Build history of the part. All positions in model axes, mm. Face numbers are marked on the shaded views. A direction names the side the tool comes from. Give positions to 0.01 mm unless a question says otherwise; leave off trailing zeros. Loops run counter-clockwise (first coordinate to the right, second up) from the corner with the lowest first, then second, coordinate; pieces in that order, holes last. Notation, with made-up numbers: (82.25, -17.5) -> (141.25, -17.5) arc R26 ccw to (141.25, 3.5) -> close; hole circle Ø2 at (-32, 78). An arc over 180 degrees is marked (long way). Answer as a JSON object with one key per item and string values. Group by question number.
Q1. Band-saw the part on B-B, the plane z = 0. Write the cut outline in (x, y).
Q2. Drop flat-ended pins along their axis: pin 1 (4 mm diameter, centred on x = 1, y = 27, fed in from -Z); pin 2 (4 mm diameter, centred on x = -8, z = -1.5, fed in from +Y); pin 3 (2 mm diameter, centred on y = 14, z = 1.5, fed in from +X); pin 4 (2.5 mm diameter, centred on y = 14, z = 0.5, fed in from -X). Give the stop position or say it passes through.
Q3. Two-plate mould, pull along X, no slides. Class the marked faces 1, 2 and 3: pulls with the +X half, pulls with the -X half, needs draft (parallel to the pull), parting line crosses it, or undercut.
Q4. Tool access for the marked faces 4, 5 and 6: list every direction of +Z, -Z, +X, -X, +Y, -Y with a clear straight run to the whole face (end or side of a thin tool).
Q5. Band-saw the part on A-A, the plane x = 0. Write the cut outline in (y, z), plus the area to 3 significant figures.
Q6. Wall check: probe 1 along Z at (x, y) = (0, 40); probe 2 along X at (y, z) = (6.5, 7.75); probe 3 along Z at (x, y) = (-11.25, 15). Give the ranges that are in metal, low to high. Write a range as from..to.
from build123d import *

# Parameters (mm, degrees)
F1_DEPTH = 50.8
F2_R     = 2.6035
F3_DEPTH = 50.801


with BuildPart() as f1:
    # F0 (on Front) → F1 (new body)
    with BuildSketch(Plane.XZ):
        with BuildLine():
            Line((-4.5085, 0), (0, 0))
            Line((0, 0), (0, 4.5085))
            Line((0, 4.5085), (-2.54, 4.5085))
            ThreePointArc((-2.54, 4.5085), (-2.957967, 4.591639), (-3.312302, 4.828398))
            Line((-3.312302, 4.828398), (-7.109602, 8.625698))
            ThreePointArc((-7.109602, 8.625698), (-7.346361, 9.815967), (-6.3373, 10.4902))
            Line((-6.3373, 10.4902), (-4.3307, 10.4902))
            ThreePointArc((-4.3307, 10.4902), (-3.558398, 10.810098), (-3.2385, 11.5824))
            Line((-3.2385, 11.5824), (-3.2385, 11.6078))
            ThreePointArc((-3.2385, 11.6078), (-3.558398, 12.380102), (-4.3307, 12.7))
            Line((-4.3307, 12.7), (-11.6078, 12.7))
            ThreePointArc((-11.6078, 12.7), (-12.380102, 12.380102), (-12.7, 11.6078))
            Line((-12.7, 11.6078), (-12.7, 4.3434))
            ThreePointArc((-12.7, 4.3434), (-12.380102, 3.571098), (-11.6078, 3.2512))
            Line((-11.6078, 3.2512), (-11.5824, 3.2512))
            ThreePointArc((-11.5824, 3.2512), (-10.810098, 3.571098), (-10.4902, 4.3434))
            Line((-10.4902, 4.3434), (-10.4902, 6.244363))
            ThreePointArc((-10.4902, 6.244363), (-9.815967, 7.253424), (-8.625698, 7.016665))
            Line((-8.625698, 7.016665), (-4.828398, 3.219365))
            ThreePointArc((-4.828398, 3.219365), (-4.591639, 2.86503), (-4.5085, 2.447063))
            Line((-4.5085, 2.447063), (-4.5085, 0))
        make_face()
        with BuildLine():
            Line((0, 4.5085), (0, 0))
            Line((0, 0), (4.5085, 0))
            Line((4.5085, 0), (4.5085, 2.447063))
            ThreePointArc((4.5085, 2.447063), (4.591639, 2.86503), (4.828398, 3.219365))
            Line((4.828398, 3.219365), (8.625698, 7.016665))
            ThreePointArc((8.625698, 7.016665), (9.815967, 7.253424), (10.4902, 6.244363))
            Line((10.4902, 6.244363), (10.4902, 4.3434))
            ThreePointArc((10.4902, 4.3434), (10.810098, 3.571098), (11.5824, 3.2512))
            Line((11.5824, 3.2512), (11.6078, 3.2512))
            ThreePointArc((11.6078, 3.2512), (12.380102, 3.571098), (12.7, 4.3434))
            Line((12.7, 4.3434), (12.7, 11.6078))
            ThreePointArc((12.7, 11.6078), (12.380102, 12.380102), (11.6078, 12.7))
            Line((11.6078, 12.7), (4.3307, 12.7))
            ThreePointArc((4.3307, 12.7), (3.558398, 12.380102), (3.2385, 11.6078))
            Line((3.2385, 11.6078), (3.2385, 11.5824))
            ThreePointArc((3.2385, 11.5824), (3.558398, 10.810098), (4.3307, 10.4902))
            Line((4.3307, 10.4902), (6.3373, 10.4902))
            ThreePointArc((6.3373, 10.4902), (7.346361, 9.815967), (7.109602, 8.625698))
            Line((7.109602, 8.625698), (3.312302, 4.828398))
            ThreePointArc((3.312302, 4.828398), (2.957967, 4.591639), (2.54, 4.5085))
            Line((2.54, 4.5085), (0, 4.5085))
        make_face()
        with BuildLine():
            Line((4.5085, 0), (0, 0))
            Line((0, 0), (0, -4.5085))
            Line((0, -4.5085), (2.54, -4.5085))
            ThreePointArc((2.54, -4.5085), (2.957967, -4.591639), (3.312302, -4.828398))
            Line((3.312302, -4.828398), (7.109602, -8.625698))
            ThreePointArc((7.109602, -8.625698), (7.346361, -9.815967), (6.3373, -10.4902))
            Line((6.3373, -10.4902), (4.3307, -10.4902))
            ThreePointArc((4.3307, -10.4902), (3.558398, -10.810098), (3.2385, -11.5824))
            Line((3.2385, -11.5824), (3.2385, -11.6078))
            ThreePointArc((3.2385, -11.6078), (3.558398, -12.380102), (4.3307, -12.7))
            Line((4.3307, -12.7), (11.6078, -12.7))
            ThreePointArc((11.6078, -12.7), (12.380102, -12.380102), (12.7, -11.6078))
            Line((12.7, -11.6078), (12.7, -4.3434))
            ThreePointArc((12.7, -4.3434), (12.380102, -3.571098), (11.6078, -3.2512))
            Line((11.6078, -3.2512), (11.5824, -3.2512))
            ThreePointArc((11.5824, -3.2512), (10.810098, -3.571098), (10.4902, -4.3434))
            Line((10.4902, -4.3434), (10.4902, -6.244363))
            ThreePointArc((10.4902, -6.244363), (9.815967, -7.253424), (8.625698, -7.016665))
            Line((8.625698, -7.016665), (4.828398, -3.219365))
            ThreePointArc((4.828398, -3.219365), (4.591639, -2.86503), (4.5085, -2.447063))
            Line((4.5085, -2.447063), (4.5085, 0))
        make_face()
        with BuildLine():
            Line((0, -4.5085), (0, 0))
            Line((0, 0), (-4.5085, 0))
            Line((-4.5085, 0), (-4.5085, -2.447063))
            ThreePointArc((-4.5085, -2.447063), (-4.591639, -2.86503), (-4.828398, -3.219365))
            Line((-4.828398, -3.219365), (-8.625698, -7.016665))
            ThreePointArc((-8.625698, -7.016665), (-9.815967, -7.253424), (-10.4902, -6.244363))
            Line((-10.4902, -6.244363), (-10.4902, -4.3434))
            ThreePointArc((-10.4902, -4.3434), (-10.810098, -3.571098), (-11.5824, -3.2512))
            Line((-11.5824, -3.2512), (-11.6078, -3.2512))
            ThreePointArc((-11.6078, -3.2512), (-12.380102, -3.571098), (-12.7, -4.3434))
            Line((-12.7, -4.3434), (-12.7, -11.6078))
            ThreePointArc((-12.7, -11.6078), (-12.380102, -12.380102), (-11.6078, -12.7))
            Line((-11.6078, -12.7), (-4.3307, -12.7))
            ThreePointArc((-4.3307, -12.7), (-3.558398, -12.380102), (-3.2385, -11.6078))
            Line((-3.2385, -11.6078), (-3.2385, -11.5824))
            ThreePointArc((-3.2385, -11.5824), (-3.558398, -10.810098), (-4.3307, -10.4902))
            Line((-4.3307, -10.4902), (-6.3373, -10.4902))
            ThreePointArc((-6.3373, -10.4902), (-7.346361, -9.815967), (-7.109602, -8.625698))
            Line((-7.109602, -8.625698), (-3.312302, -4.828398))
            ThreePointArc((-3.312302, -4.828398), (-2.957967, -4.591639), (-2.54, -4.5085))
            Line((-2.54, -4.5085), (0, -4.5085))
        make_face()
    extrude(amount=-F1_DEPTH)

    # F2 (on face) → F3 (cut, through all)
    with BuildSketch(Plane.XZ):
        Circle(F2_R)
    extrude(amount=-F3_DEPTH, mode=Mode.SUBTRACT)


solid = f1.part
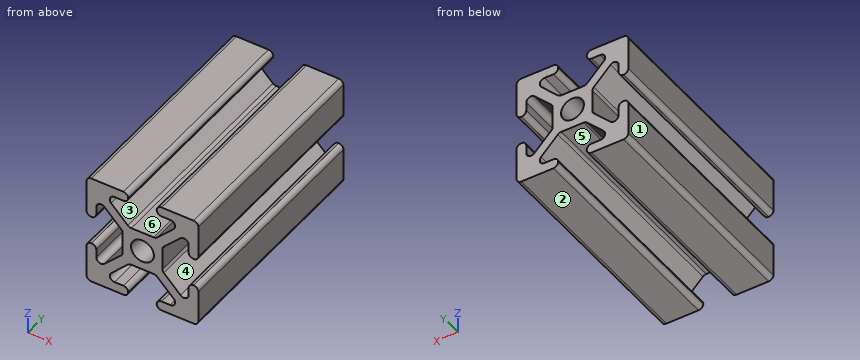
Worked answers:
{
 "1": {"outline": "(-4.51, 0) -> (-2.6, 0) -> (-2.6, 50.8) -> (-4.51, 50.8) -> close; (2.6, 0) -> (4.51, 0) -> (4.51, 50.8) -> (2.6, 50.8) -> close"},
 "2": {"pin 1": "z = -4.61", "pin 2": "through", "pin 3": "x = 4.51", "pin 4": "x = -4.51"},
 "3": {"face 1": "pulls with the -X half", "face 2": "needs draft", "face 3": "undercut"},
 "4": {"face 4": "+Y, -Y", "face 5": "-Z, +Y, -Y", "face 6": "+Z, +Y, -Y"},
 "5": {"outline": "(0, -4.51) -> (50.8, -4.51) -> (50.8, -2.6) -> (0, -2.6) -> close; (0, 2.6) -> (50.8, 2.6) -> (50.8, 4.51) -> (0, 4.51) -> close", "area": "194 mm2"},
 "6": {"probe 1": "-4.51..-2.6, 2.6..4.51", "probe 2": "-12.7..-6.23, 6.23..12.7", "probe 3": "-12.7..-3.3, 3.3..12.7"}
}
